Read the model definition and answer for the solid it produces. Units are mm, in the model's axes. Coordinates: 2 decimals unless noted, no trailing zeros. Answer as a JSON object with one key per item and string values. Group by question number.
from build123d import *

# Parameters (mm, degrees)
SKETCH1_R           = 2.1
BOSS_EXTRUDE1_DEPTH = 180.2


with BuildPart() as part:
    # Sketch1 → Boss-Extrude1 (new, symmetric)
    with BuildSketch(Plane.XY):
        with BuildLine():
            Line((4.58, -20), (9.5, -20))
            ThreePointArc((9.5, -20), (9.853553391, -19.853553391), (10, -19.5))
            Line((10, -19.5), (10, -14.58))
            Line((10, -14.58), (8.545, -13.125))
            Line((8.545, -13.125), (8.2, -13.125))
            Line((8.2, -13.125), (8.2, -15.5))
            Line((8.2, -15.5), (6.560660172, -15.5))
            Line((6.560660172, -15.5), (3.9, -12.839339828))
            Line((3.9, -12.839339828), (3.9, -10.21))
            Line((3.9, -10.21), (3.69, -10))
            Line((3.69, -10), (3.9, -9.79))
            Line((3.9, -9.79), (3.9, -7.160660172))
            Line((3.9, -7.160660172), (6.560660172, -4.5))
            Line((6.560660172, -4.5), (8.2, -4.5))
            Line((8.2, -4.5), (8.2, -6.875))
            Line((8.2, -6.875), (8.545, -6.875))
            Line((8.545, -6.875), (10, -5.42))
            Line((10, -5.42), (10, 5.42))
            Line((10, 5.42), (8.545, 6.875))
            Line((8.545, 6.875), (8.2, 6.875))
            Line((8.2, 6.875), (8.2, 4.5))
            Line((8.2, 4.5), (6.560660172, 4.5))
            Line((6.560660172, 4.5), (3.9, 7.160660172))
            Line((3.9, 7.160660172), (3.9, 9.79))
            Line((3.9, 9.79), (3.69, 10))
            Line((3.69, 10), (3.9, 10.21))
            Line((3.9, 10.21), (3.9, 12.839339828))
            Line((3.9, 12.839339828), (6.560660172, 15.5))
            Line((6.560660172, 15.5), (8.2, 15.5))
            Line((8.2, 15.5), (8.2, 13.125))
            Line((8.2, 13.125), (8.545, 13.125))
            Line((8.545, 13.125), (10, 14.58))
            Line((10, 14.58), (10, 19.5))
            ThreePointArc((10, 19.5), (9.853553391, 19.853553391), (9.5, 20))
            Line((9.5, 20), (4.58, 20))
            Line((4.58, 20), (3.125, 18.545))
            Line((3.125, 18.545), (3.125, 18.2))
            Line((3.125, 18.2), (5.5, 18.2))
            Line((5.5, 18.2), (5.5, 16.560660172))
            Line((5.5, 16.560660172), (2.839339828, 13.9))
            Line((2.839339828, 13.9), (0.21, 13.9))
            Line((0.21, 13.9), (0, 13.69))
            Line((0, 13.69), (-0.21, 13.9))
            Line((-0.21, 13.9), (-2.839339828, 13.9))
            Line((-2.839339828, 13.9), (-5.5, 16.560660172))
            Line((-5.5, 16.560660172), (-5.5, 18.2))
            Line((-5.5, 18.2), (-3.125, 18.2))
            Line((-3.125, 18.2), (-3.125, 18.545))
            Line((-3.125, 18.545), (-4.58, 20))
            Line((-4.58, 20), (-9.5, 20))
            ThreePointArc((-9.5, 20), (-9.853553391, 19.853553391), (-10, 19.5))
            Line((-10, 19.5), (-10, 14.58))
            Line((-10, 14.58), (-8.545, 13.125))
            Line((-8.545, 13.125), (-8.2, 13.125))
            Line((-8.2, 13.125), (-8.2, 15.5))
            Line((-8.2, 15.5), (-6.560660172, 15.5))
            Line((-6.560660172, 15.5), (-3.9, 12.839339828))
            Line((-3.9, 12.839339828), (-3.9, 10.21))
            Line((-3.9, 10.21), (-3.69, 10))
            Line((-3.69, 10), (-3.9, 9.79))
            Line((-3.9, 9.79), (-3.9, 7.160660172))
            Line((-3.9, 7.160660172), (-6.560660172, 4.5))
            Line((-6.560660172, 4.5), (-8.2, 4.5))
            Line((-8.2, 4.5), (-8.2, 6.875))
            Line((-8.2, 6.875), (-8.545, 6.875))
            Line((-8.545, 6.875), (-10, 5.42))
            Line((-10, 5.42), (-10, -5.42))
            Line((-10, -5.42), (-8.545, -6.875))
            Line((-8.545, -6.875), (-8.2, -6.875))
            Line((-8.2, -6.875), (-8.2, -4.5))
            Line((-8.2, -4.5), (-6.560660172, -4.5))
            Line((-6.560660172, -4.5), (-3.9, -7.160660172))
            Line((-3.9, -7.160660172), (-3.9, -9.79))
            Line((-3.9, -9.79), (-3.69, -10))
            Line((-3.69, -10), (-3.9, -10.21))
            Line((-3.9, -10.21), (-3.9, -12.839339828))
            Line((-3.9, -12.839339828), (-6.560660172, -15.5))
            Line((-6.560660172, -15.5), (-8.2, -15.5))
            Line((-8.2, -15.5), (-8.2, -13.125))
            Line((-8.2, -13.125), (-8.545, -13.125))
            Line((-8.545, -13.125), (-10, -14.58))
            Line((-10, -14.58), (-10, -19.5))
            ThreePointArc((-10, -19.5), (-9.853553391, -19.853553391), (-9.5, -20))
            Line((-9.5, -20), (-4.58, -20))
            Line((-4.58, -20), (-3.125, -18.545))
            Line((-3.125, -18.545), (-3.125, -18.2))
            Line((-3.125, -18.2), (-5.5, -18.2))
            Line((-5.5, -18.2), (-5.5, -16.560660172))
            Line((-5.5, -16.560660172), (-2.839339828, -13.9))
            Line((-2.839339828, -13.9), (-0.21, -13.9))
            Line((-0.21, -13.9), (0, -13.69))
            Line((0, -13.69), (0.21, -13.9))
            Line((0.21, -13.9), (2.839339828, -13.9))
            Line((2.839339828, -13.9), (5.5, -16.560660172))
            Line((5.5, -16.560660172), (5.5, -18.2))
            Line((5.5, -18.2), (3.125, -18.2))
            Line((3.125, -18.2), (3.125, -18.545))
            Line((3.125, -18.545), (4.58, -20))
        make_face()
        with Locations((0, -10)):
            Circle(SKETCH1_R, mode=Mode.SUBTRACT)
        Polygon((-6.239339828, -2.7), (-8.2, -2.7), (-8.2, 2.7), (-6.239339828, 2.7), (-2.839339828, 6.1), (2.839339828, 6.1), (6.239339828, 2.7), (8.2, 2.7), (8.2, -2.7), (6.239339828, -2.7), (2.839339828, -6.1), (-2.839339828, -6.1), align=None, mode=Mode.SUBTRACT)
        with Locations((0, 10)):
            Circle(SKETCH1_R, mode=Mode.SUBTRACT)
    extrude(amount=BOSS_EXTRUDE1_DEPTH, both=True)


solid = part.part
1. A cutting plane is placed at A-A on z = 150.5. State how many separate pieces and enclosed holes the cut face has, and give its area (3 significant figures).
2. Given pin 1 (0.8 mm diameter, centred on x = 1.5, z = 9.5, fed in from +Y); pin 2 (6 mm diameter, centred on x = -0.5, z = 10, fed in from -Y); pin 3 (0.8 mm diameter, centred on y = -8.5, z = 69.5, fed in from -X), each flat-ended and moving along its own axis, determine where each tip first touches the part or whether it passes through.
3. For a pull along Y with two mould halves and no side action, classify faces 1 (the flat face through (-5, 5, 180.2)), 2 (the flat face through (0, -6.1, 3)), 3 (the flat face through (0, 6.1, 3)) as pulls with the +Y half, pulls with the -Y half, needs draft (parallel to the pull), parting line crosses it, or undercut.
4. Straight lines are drawn through the part: L1, parallel to Y at x = -7, z = -94.5; L2, parallel to Y at x = -0.5, z = -93; L3, parallel to X at y = 2, z = 37.5. For each, find the intervals that lie inside material, in ascending order.
Derived:
{
 "1": {"separate pieces": "1", "enclosed holes": "3", "area": "300 mm2"},
 "2": {"pin 1": "stops at y = 13.9", "pin 2": "stops at y = -18.92", "pin 3": "stops at x = -3.9"},
 "3": {"face 1": "needs draft", "face 2": "undercut", "face 3": "undercut"},
 "4": {"L1": "y = -20 to -15.5, -4.5 to -2.7, 2.7 to 4.5, 15.5 to 20", "L2": "y = -13.9 to -12.04, -7.96 to -6.1, 6.1 to 7.96, 12.04 to 13.9", "L3": "x = -10 to -8.2, 8.2 to 10"}
}
